Can you work these out from the model? Positions are in its coordinate system, mm. A direction names the side the tool comes from. Give positions to 0.01 mm unless a question says otherwise; leave off trailing zeros. Loops run counter-clockwise (first coordinate to the right, second up) from the corner with the lowest first, then second, coordinate; pieces in that order, holes last. Notation, with made-up numbers: M -5,-16 L 47,-16 A17 ccw 47,2 Z; hole C 8,48.5 d2. An arc over 180 degrees is marked long. Answer as a JSON object with one key per item and string values.
```python
from build123d import *

# Parameters (mm, degrees)
SKETCH1_R           = 15
SKETCH1_R_2         = 10
BOSS_EXTRUDE1_DEPTH = 21
SKETCH2_R           = 3.5
CUT_EXTRUDE1_DEPTH  = 60
FILLET1_R           = 8
SKETCH5_R           = 10
BOSS_EXTRUDE2_DEPTH = 6.5
BOSS_EXTRUDE3_DEPTH = 9
SKETCH6_R           = 12.5
BOSS_EXTRUDE4_DEPTH = 40
BOSS_EXTRUDE5_DEPTH = 4
SKETCH1_3_R         = 10
CUT_EXTRUDE2_DEPTH  = 21
SKETCH10_W          = 19
SKETCH10_H          = 38
SKETCH11_W          = 38
SKETCH11_H          = 38
CUT_EXTRUDE3_DEPTH  = 51


with BuildPart() as part:
    # Sketch1 → Boss-Extrude1 (new body, symmetric)
    with BuildSketch(Plane.XY):
        with BuildLine():
            ThreePointArc((22, 0), (0, 22), (-22, 0))
            Line((-22, 0), (-22, -43))
            Line((-22, -43), (-48, -43))
            Line((-48, -43), (-48, -50))
            Line((-48, -50), (-16, -50))
            ThreePointArc((-16, -50), (0, -34), (16, -50))
            Line((16, -50), (48, -50))
            Line((48, -50), (48, -43))
            Line((48, -43), (22, -43))
            Line((22, -43), (22, 0))
        make_face()
        Circle(SKETCH1_R, mode=Mode.SUBTRACT)
        with BuildLine():
            ThreePointArc((16, -50), (0, -34), (-16, -50))
            Line((-16, -50), (-10, -50))
            ThreePointArc((-10, -50), (0, -40), (10, -50))
            Line((10, -50), (16, -50))
        make_face()
        Circle(SKETCH1_R)
        Circle(SKETCH1_R_2, mode=Mode.SUBTRACT)
    extrude(amount=BOSS_EXTRUDE1_DEPTH, both=True)

    # Sketch2 → Cut-Extrude1 (cut)
    with BuildSketch(Plane(origin=(0, -43, 0), x_dir=(1, 0, 0), z_dir=(0, 1, 0))):
        with Locations((40, 13.5)):
            Circle(SKETCH2_R)
        with Locations((40, -13.5)):
            Circle(SKETCH2_R)
    cut_extrude1 = extrude(amount=-CUT_EXTRUDE1_DEPTH, mode=Mode.SUBTRACT)

    # Mirror1: Cut-Extrude1 across plane
    add(cut_extrude1.mirror(Plane(origin=(0, 0, 0), x_dir=(0, 0, 1), z_dir=(1, 0, 0))), mode=Mode.SUBTRACT)

    # Fillet1
    fillet1_edges = [part.edges().sort_by_distance(p)[0] for p in [
        (-48, -46.5, -21),
        (48, -46.5, -21),
        (48, -46.5, 21),
        (-48, -46.5, 21),
    ]]
    fillet(fillet1_edges, radius=FILLET1_R)

    # Sketch5 → Boss-Extrude2 (add)
    with BuildSketch(Plane.XY.offset(21)):
        with BuildLine():
            Line((-3.053517872, -14.68591259), (-3.053517872, -34.294076639))
            ThreePointArc((-3.053517872, -34.294076639), (-0.054484182, -34.000092767), (2.946482128, -34.273644953))
            Line((2.946482128, -34.273644953), (2.946482128, -14.707761321))
            ThreePointArc((2.946482128, -14.707761321), (0.054621464, 14.99990055), (-3.053517872, -14.68591259))
        make_face()
        Circle(SKETCH5_R, mode=Mode.SUBTRACT)
    boss_extrude2 = extrude(amount=BOSS_EXTRUDE2_DEPTH)

    # Sketch5<3> → Boss-Extrude3 (add)
    with BuildSketch(Plane.XY.offset(21)):
        with BuildLine():
            ThreePointArc((-3.053517872, -34.294076639), (-12.346179286, -39.822974058), (-16, -50))
            Line((-16, -50), (-10, -50))
            ThreePointArc((-10, -50), (0, -40), (10, -50))
            Line((10, -50), (16, -50))
            ThreePointArc((16, -50), (12.311452271, -39.780991096), (2.946482128, -34.273644953))
            ThreePointArc((2.946482128, -34.273644953), (-0.054484182, -34.000092767), (-3.053517872, -34.294076639))
        make_face()
    boss_extrude3 = extrude(amount=BOSS_EXTRUDE3_DEPTH)

    # Mirror2: Boss-Extrude2, Boss-Extrude3 across plane
    add(boss_extrude2.mirror(Plane.XY))
    add(boss_extrude3.mirror(Plane.XY))

    # Sketch6 → Boss-Extrude4 (add)
    with BuildSketch(Plane(origin=(0, 0, 0), x_dir=(0, 0, -1), z_dir=(1, 0, 0))):
        Circle(SKETCH6_R)
    boss_extrude4 = extrude(amount=BOSS_EXTRUDE4_DEPTH)

    # Sketch7 → Boss-Extrude5 (add, symmetric)
    with BuildSketch(Plane.XY):
        Polygon((22, -43), (48, -43), (36, -10.955283754), (22, -10.955283754), align=None)
    boss_extrude5 = extrude(amount=BOSS_EXTRUDE5_DEPTH, both=True)

    # Sketch1<3> → Cut-Extrude2 (cut, symmetric)
    with BuildSketch(Plane.XY):
        Circle(SKETCH1_3_R)
    cut_extrude2 = extrude(amount=CUT_EXTRUDE2_DEPTH, both=True, mode=Mode.SUBTRACT)

    # Sketch8 → Cut-Revolve1 (revolve, cut)
    with BuildSketch(Plane(origin=(0, 0, 0), x_dir=(1, 0, 0), z_dir=(0, 1, 0))):
        Polygon((40, 0), (22, 0), (23.87378357, 4.5), (24.87378357, 4.5), (24.87378357, 5), (40, 5), align=None)
    cut_revolve1 = revolve(axis=Axis((40, 0, 0), (-1, 0, 0)), mode=Mode.SUBTRACT)

    # Mirror4: Boss-Extrude4, Boss-Extrude5, Cut-Extrude2, Cut-Revolve1 across plane
    add(boss_extrude4.mirror(Plane(origin=(0, 0, 0), x_dir=(0, 0, 1), z_dir=(1, 0, 0))))
    add(boss_extrude5.mirror(Plane(origin=(0, 0, 0), x_dir=(0, 0, 1), z_dir=(1, 0, 0))))
    add(cut_extrude2.mirror(Plane(origin=(0, 0, 0), x_dir=(0, 0, 1), z_dir=(1, 0, 0))), mode=Mode.SUBTRACT)
    add(cut_revolve1.mirror(Plane(origin=(0, 0, 0), x_dir=(0, 0, 1), z_dir=(1, 0, 0))), mode=Mode.SUBTRACT)

    # Sketch10 → Cut-Revolve2 (revolve, cut)
    with BuildSketch(Plane(origin=(0, 0, 0), x_dir=(1, 0, 0), z_dir=(0, 1, 0))):
        with Locations((-9.5, 0)):
            Rectangle(SKETCH10_W, SKETCH10_H)
    revolve(axis=Axis((0, 0, -19), (0, 0, 1)), mode=Mode.SUBTRACT)

    # Sketch11 → Cut-Extrude3 (cut, through all)
    with BuildSketch(Plane(origin=(0, 0, 0), x_dir=(1, 0, 0), z_dir=(0, 1, 0))):
        Rectangle(SKETCH11_W, SKETCH11_H)
    extrude(amount=-CUT_EXTRUDE3_DEPTH, mode=Mode.SUBTRACT)


solid = part.part
```
1) Will these pins go through, and if not, where does the flat tip stop? pin 1 Ø6 at (x, y) = (-29.5, 2.5) entering from +Z; pin 2 Ø6 at (y, z) = (-23.5, 23.5) entering from -X; pin 3 Ø7 at (y, z) = (-25, 25) entering from +X.
Answer list:
{"pin 1": "z = 12.5", "pin 2": "x = -22", "pin 3": "x = 2.95"}
2) Suppose I cut it at A-A, the plane x = 0. Write out the boundary of the cut face in (y, z).
Answer list:
{"outline": "M -40,-30 L -34,-30 L -34,-27.5 L -10,-27.5 L -10,-19 L -40,-19 Z; M -40,19 L -10,19 L -10,27.5 L -34,27.5 L -34,30 L -40,30 Z; M 10,-27.5 L 15,-27.5 L 15,-21 L 22,-21 L 22,21 L 15,21 L 15,27.5 L 10,27.5 L 10,19 L 19,19 L 19,-19 L 10,-19 Z"}
3) Please list where these lines run through material, in increasing order: line 1 along X through (y, z) = (-48, -13.5); line 2 along Z through (x, y) = (24.15, 0); line 3 along X through (y, z) = (0, -23.5). Write a range as from..to.
Answer list:
{"line 1": "-47.98..-43.5, -36.5..-19, 19..36.5, 43.5..47.98", "line 2": "-12.5..-4.5, 4.5..12.5", "line 3": "-15..-10, 10..15"}
4) For faces 5 (the cylindrical face through (0, 19, 0)), 6 (the flat face through (35, -43, 13)), 7 (the cylindrical face through (24.38, -4.46, 0.59)), which set-ups out of +Z, -Z, +X, -X, +Y, -Y let a thin tool reach every point of the face, with its end or its side?
Answer list:
{"face 5": "-Y", "face 6": "+Z, +X", "face 7": "+X"}
5) Suppose I cut it at B-B, the plane x = 27. Write out the boundary of the cut face in (y, z), and give its area (3 significant figures).
Answer list:
{"outline": "M -50,-21 L -43,-21 L -43,-4 L -11.84,-4 A12.5 ccw long -11.84,4 L -43,4 L -43,21 L -50,21 Z; hole C 0,0 d10", "area": "952 mm^2"}
6) Suppose I cut it at C-C, the plane y = -26. Write out the boundary of the cut face in (x, z), and give its area (3 significant figures).
Answer list:
{"outline": "M -41.63,-4 L -22,-4 L -22,-21 L -3.05,-21 L -3.05,-27.5 L 2.95,-27.5 L 2.95,-21 L 22,-21 L 22,-4 L 41.63,-4 L 41.63,4 L 22,4 L 22,21 L 2.95,21 L 2.95,27.5 L -3.05,27.5 L -3.05,21 L -22,21 L -22,4 L -41.63,4 Z; hole M -19,-19 L 19,-19 L 19,19 L -19,19 Z", "area": "796 mm^2"}
7) If we mould it in two halves opening along Z, with no side actions, what happens to faces 1 (the flat face through (-19, -25, 0)), 2 (the cylindrical face through (31.331, 12.394, 1.627)), 3 (the cylindrical face through (-37.2, -46.5, -11.4)), 4 (the cylindrical face through (0, -40, -24))? For each: +Z half, -Z half, draft (parallel to the pull), parting line (faces both ways), or undercut.
Answer list:
{"face 1": "undercut", "face 2": "parting line", "face 3": "undercut", "face 4": "draft"}
